Model file for the job. Use its own axes, mm. Face numbers are marked on the shaded views. A direction names the side the tool comes from. Round coordinates to 2 decimals unless told otherwise and drop trailing zeros. Order: outer loops, then holes, each group sorted by start corner. A loop starts at its lowest first (then second) coordinate and runs counter-clockwise, first axis right, second up. Notation, with made-up numbers: M 6.5,76 L 54.5,76 A20 cw 54.5,85 Z; hole C 76.25,-6 d9. An arc over 180 degrees is marked long. Return JSON: item names as keys, results as strings. Group by question number.
Item 1: Slice it at A-A on z = -58. Write the cut outline in (x, y).
Item 2: Probe line 1 along Z through (x, y) = (-11.75, 5.25); line 2 along Y through (x, z) = (-11.2, -58); line 3 along Z through (x, y) = (-10.5, 6). List the from-to ranges inside material, lowest first.
Item 3: Slice it at D-D on y = 8. Write the cut outline in (x, z), then the cut area to 3 significant figures.
Item 4: Pin check, flat tips, straight feed: pin 1 Ø6 at (x, y) = (-2, 5) entering from +Z; pin 2 Ø4 at (y, z) = (2.5, -8.5) entering from +X; pin 3 Ø5 at (x, y) = (-5, 1.5) entering from -Z. Stop position of each tip, or through.
Item 5: Slice it at C-C on x = -10.75. Write the cut outline in (y, z), then the cut area to 3 significant figures.
Item 6: Which spindle directions (+Z, -Z, +X, -X, +Y, -Y) get a long thin tool onto all of the face, cutting with end or side? Do the marked faces 1, 2 and 3. Say none if no direction does.
Item 7: Slice it at B-B on y = 5. Write the cut outline in (x, z).
Autodesk Inventor part; units mm, degrees
ref_plane "YZ Plane" through (0, 0, 0) normal (1, 0, 0) x (0, 1, 0)
ref_plane "XZ Plane" through (0, 0, 0) normal (0, 1, 0) x (-1, 0, 0)
ref_plane "XY Plane" through (0, 0, 0) normal (0, 0, 1) x (1, 0, 0)
sketch "Sketch1" plane through (0, 0, 0) normal (0, 1, 0) x (-1, 0, 0)
  line L0 (0, 0) -> (10, 0)
  line L1 (10, 0) -> (10, 10)
  line L2 (10, 10) -> (15, 10)
  line L3 (15, 10) -> (15, -63)
  line L4 (15, -63) -> (10, -63)
  line L5 (10, -63) -> (10, -53)
  line L6 (10, -53) -> (0, -53)
  line L7 (0, -53) -> (0, 0)
  dimension "d6" = 53
  dimension "d7" = 73
  dimension "d8" = 10
  dimension "d9" = 5
  dimension "d10" = 10
extrude "Extrusion1" add sketch "Sketch1" along normal blind 10
hole "Hole1" at (-10, 5, 5) direction (-1, 0, 0) diameter 4.2 end through all
hole "Hole2" at (-10, 5, -58) direction (-1, 0, 0) diameter 4.2 end through all
properties part number "frontBeam" material "ABS Plastic"
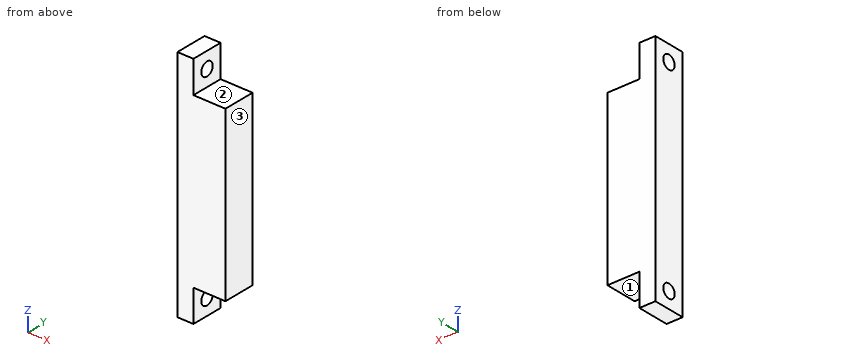
Output values:
{
 "1": {"outline": "M -15,0 L -10,0 L -10,2.9 L -15,2.9 Z; M -15,7.1 L -10,7.1 L -10,10 L -15,10 Z"},
 "2": {"line 1": "-63 to -60.09, -55.91 to 2.91, 7.09 to 10", "line 2": "0 to 2.9, 7.1 to 10", "line 3": "-63 to -59.85, -56.15 to 3.15, 6.85 to 10"},
 "3": {"outline": "M -15,-63 L -10,-63 L -10,-53 L 0,-53 L 0,0 L -10,0 L -10,10 L -15,10 Z", "area": "895 mm²"},
 "4": {"pin 1": "z = 0", "pin 2": "x = 0", "pin 3": "z = -53"},
 "5": {"outline": "M 0,-63 L 10,-63 L 10,10 L 0,10 Z; hole C 5,-58 d4.2; hole C 5,5 d4.2", "area": "702 mm²"},
 "6": {"face 1": "-Z, +X, +Y, -Y", "face 2": "+Z, +X, +Y, -Y", "face 3": "+Z, -Z, +X, +Y, -Y"},
 "7": {"outline": "M -15,-63 L -10,-63 L -10,-60.1 L -15,-60.1 Z; M -15,-55.9 L -10,-55.9 L -10,-53 L 0,-53 L 0,0 L -10,0 L -10,2.9 L -15,2.9 Z; M -15,7.1 L -10,7.1 L -10,10 L -15,10 Z"}
}
